from build123d import *

# Parameters (mm, degrees)
SKETCH1_W               = 60
SKETCH1_H               = 69.5
BOSS_EXTRUDE1_DEPTH     = 4.75
SKETCH2_W               = 10
SKETCH2_H               = 4.75
CUT_EXTRUDE1_DEPTH      = 1
CUT_EXTRUDE1_DEPTH_BACK = 5.75
SKETCH3_R               = 1.5
CUT_EXTRUDE2_DEPTH      = 1
CUT_EXTRUDE2_DEPTH_BACK = 5.75


with BuildPart() as part:
    # Sketch1 → Boss-Extrude1 (new body)
    with BuildSketch(Plane.XY):
        Rectangle(SKETCH1_W, SKETCH1_H)
    extrude(amount=BOSS_EXTRUDE1_DEPTH)

    # Sketch2 → Cut-Extrude1 (cut, two sides)
    with BuildSketch(Plane.XY.offset(4.75)) as cut_extrude1_sk:
        with Locations((-25, 32.375)):
            Rectangle(SKETCH2_W, SKETCH2_H)
        with Locations((-25, -32.375)):
            Rectangle(SKETCH2_W, SKETCH2_H)
        with Locations((25, -32.375)):
            Rectangle(SKETCH2_W, SKETCH2_H)
        with Locations((25, 32.375)):
            Rectangle(SKETCH2_W, SKETCH2_H)
    extrude(amount=CUT_EXTRUDE1_DEPTH, mode=Mode.SUBTRACT)
    extrude(cut_extrude1_sk.sketch, amount=-CUT_EXTRUDE1_DEPTH_BACK, mode=Mode.SUBTRACT)

    # Sketch3 → Cut-Extrude2 (cut, two sides)
    with BuildSketch(Plane.XY.offset(4.75)) as cut_extrude2_sk:
        with Locations((-15, 12)):
            Circle(SKETCH3_R)
        with Locations((-15, -12)):
            Circle(SKETCH3_R)
        with Locations((15, -12)):
            Circle(SKETCH3_R)
        with Locations((15, 12)):
            Circle(SKETCH3_R)
    extrude(amount=CUT_EXTRUDE2_DEPTH, mode=Mode.SUBTRACT)
    extrude(cut_extrude2_sk.sketch, amount=-CUT_EXTRUDE2_DEPTH_BACK, mode=Mode.SUBTRACT)


solid = part.part
Can you work these out from the model? Positions are in its coordinate system, mm. A direction names the side the tool comes from. Coordinates: 2 decimals unless noted, no trailing zeros. Write each loop counter-clockwise with the first axis right and the second up, starting at its lowest first coordinate (ties: lowest second). Pieces come first, ordered by that corner, then holes. Notation, with made-up numbers: (-5, -16.5) -> (34, -16.5) arc R11 ccw to (34, -1.5) -> close; hole circle Ø8 at (0.5, 35). An arc over 180 degrees is marked (long way). Write each question's results on one line, items separated by ' | '. Start each with the question number.
Q1. If I drill on probe 1 along Y at (x, z) = (15, 3.05); probe 2 along X at (y, z) = (-30.5, 2.15); probe 3 along Y at (x, z) = (-15.5, 1.25), over which ranges is the centre line in solid material (lowest first)?
Q2. Imagine slicing it at B-B (x = 15). Write out the boundary of the cut face in (y, z).
Q3. Imagine slicing it at C-C (x = 26). Write out the boundary of the cut face in (y, z).
Q4. On a 3-axis mill with a long thin cutter (end or side, diameter ignored), from which of +Z, -Z, +X, -X, +Y, -Y can I reach the whole of each face in a straight line? I mean faces 4 (the face through (25, -30, 2)), 5 (the face through (-20, 32, 2)), 6 (the face through (-25, -30, 2)), 7 (the face through (20, 32, 2)). Say none if no direction works.
Q5. We'd pull the mould along X, two halves only. Please class faces 1 (the face through (0, 34.75, 2)), 2 (the face through (13.5, 12.07, 2.41)), 3 (the face through (-30, 0, 2)): +X half, -X half, draft (parallel to the pull), parting line (faces both ways), or undercut.
Q6. I'm going to push flat-ended pins straight in: pin 1 (2.5 mm diameter, centred on x = 24, z = 2, fed in from -Y); pin 2 (2.5 mm diameter, centred on y = 32, z = 1, fed in from -X); pin 3 (1.4 mm diameter, centred on y = -33, z = 2.5, fed in from +X). Where does each tip first touch, or does it pass through?
Q7. Imagine slicing it at A-A (y = -12). Write out the boundary of the cut face in (x, z), then the cut area to 4 significant figures.
Taken from the geometry:
1) probe 1: y = -34.75 to -13.5, -10.5 to 10.5, 13.5 to 34.75 | probe 2: x = -20 to 20 | probe 3: y = -34.75 to -13.41, -10.59 to 10.59, 13.41 to 34.75
2) outline: (-34.75, 0) -> (-13.5, 0) -> (-13.5, 4.75) -> (-34.75, 4.75) -> close; (-10.5, 0) -> (10.5, 0) -> (10.5, 4.75) -> (-10.5, 4.75) -> close; (13.5, 0) -> (34.75, 0) -> (34.75, 4.75) -> (13.5, 4.75) -> close
3) outline: (-30, 0) -> (30, 0) -> (30, 4.75) -> (-30, 4.75) -> close
4) face 4: +Z, -Z, +X, -Y | face 5: +Z, -Z, -X, +Y | face 6: +Z, -Z, -X, -Y | face 7: +Z, -Z, +X, +Y
5) face 1: draft | face 2: undercut | face 3: -X half
6) pin 1: stops at y = -30 | pin 2: stops at x = -20 | pin 3: stops at x = 20
7) outline: (-30, 0) -> (-16.5, 0) -> (-16.5, 4.75) -> (-30, 4.75) -> close; (-13.5, 0) -> (13.5, 0) -> (13.5, 4.75) -> (-13.5, 4.75) -> close; (16.5, 0) -> (30, 0) -> (30, 4.75) -> (16.5, 4.75) -> close | area: 256.5 mm^2
